For this review, take the finished solid that the model builds, in its own axes (mm). A direction names the side the tool comes from. Round coordinates to 2 decimals unless told otherwise and drop trailing zeros. Loops run counter-clockwise (first coordinate to the right, second up) from the corner with the lowest first, then second, coordinate; pieces in that order, holes last. Notation, with made-up numbers: (41, 28.25) -> (49, 28.25) arc R24 cw to (49, 50.25) -> close; hole circle Ø11 at (21, 78.5). An arc over 180 degrees is marked (long way). One line per question, with ' | ' between items. Start each with the question number.
1. Wall thickness on line 1 along Y through (x, z) = (0, 6.5) (3 decimals); line 2 along Y through (x, z) = (5, 25); line 3 along X through (y, z) = (33, 27.5): over which ranges is each line inside the solid? List them lowest first.
2. For pin 1 Ø10 at (x, y) = (23, 22.5) entering from -Z; pin 2 Ø2 at (x, z) = (-38.5, 24.5) entering from -Y; pin 3 Ø2 at (x, z) = (-41, 23) entering from +Y; pin 4 Ø8 at (y, z) = (-31, 8) entering from -X, all flat-tipped, find the tip position at first contact; note any pin that passes through.
3. Draft analysis for pull direction X (two halves, no side actions). For faces 1 (the face through (-40, 0, 23)), 2 (the face through (-23.977, 1.055, 4.056)), 3 (the face through (24.2, 0.5, 8)), state which applies: pulls with the +X half, pulls with the -X half, needs draft (parallel to the pull), parting line crosses it, or undercut.
4. Consider section C-C (y = -27). Write out the cut boundary in (x, z), and give its area (3 significant figures).
5. Consider section D-D (z = 6). Write out the cut boundary in (x, y) (3 decimals).
6. Consider section A-A (z = 33.5). Write out the cut boundary in (x, y) (3 decimals), and give its area (3 significant figures).
7. For faces 4 (the face through (-38, 14.427, 23)), 5 (the face through (18, -18, 0)), list the 3-axis set-ups (+Z, -Z, +X, -X, +Y, -Y) from which the entire face can be reached by the end or side of a thin tool; tool diameter is ignored.
```python
from build123d import *

# Parameters (mm, degrees)
SKETCH1_R           = 42.375
BOSS_EXTRUDE1_DEPTH = 8
BOSS_EXTRUDE2_DEPTH = 30
SKETCH4_R           = 24
CUT_EXTRUDE1_DEPTH  = 20


with BuildPart() as part:
    # Sketch1 → Boss-Extrude1 (new body)
    with BuildSketch(Plane.XY):
        Circle(SKETCH1_R)
    extrude(amount=BOSS_EXTRUDE1_DEPTH)

    # Sketch2 → Boss-Extrude2 (add)
    with BuildSketch(Plane.XY.offset(8)):
        with BuildLine():
            ThreePointArc((38.225, 0), (0, -38.225), (-38.225, 0))
            Line((-38.225, 0), (-42.375, 0))
            ThreePointArc((-42.375, 0), (0, -42.375), (42.375, 0))
            ThreePointArc((42.375, 0), (7.323876107, 41.737291045), (-39.843358172, 14.42731557))
            Line((-39.843358172, 14.42731557), (-35.397785106, 14.42731557))
            ThreePointArc((-35.397785106, 14.42731557), (7.35086013, 37.511537963), (38.225, 0))
        make_face()
    extrude(amount=BOSS_EXTRUDE2_DEPTH)

    # Sketch4 → Cut-Extrude1 (cut)
    with BuildSketch(Plane.XY.offset(8)):
        Circle(SKETCH4_R)
    extrude(amount=-CUT_EXTRUDE1_DEPTH, mode=Mode.SUBTRACT)


solid = part.part
```
Answer block:
1) line 1: y = -42.375 to -24, 24 to 42.375 | line 2: y = -42.08 to -37.9, 37.9 to 42.08 | line 3: x = -26.58 to -19.29, 19.29 to 26.58
2) pin 1: stops at z = 0 | pin 2: stops at y = -19.73 | pin 3: stops at y = 0 | pin 4: stops at x = -32.66
3) face 1: needs draft | face 2: undercut | face 3: undercut
4) outline: (-32.66, 0) -> (32.66, 0) -> (32.66, 38) -> (27.06, 38) -> (27.06, 8) -> (-27.06, 8) -> (-27.06, 38) -> (-32.66, 38) -> close | area: 859 mm2
5) outline: circle Ø84.75 at (0, 0); hole circle Ø48 at (0, 0)
6) outline: (-42.375, 0) arc R42.375 ccw (long way) to (-39.843, 14.427) -> (-35.398, 14.427) arc R38.225 cw (long way) to (-38.225, 0) -> close | area: 990 mm2
7) face 4: +Z, -X | face 5: -Z, +X, -X, +Y, -Y
